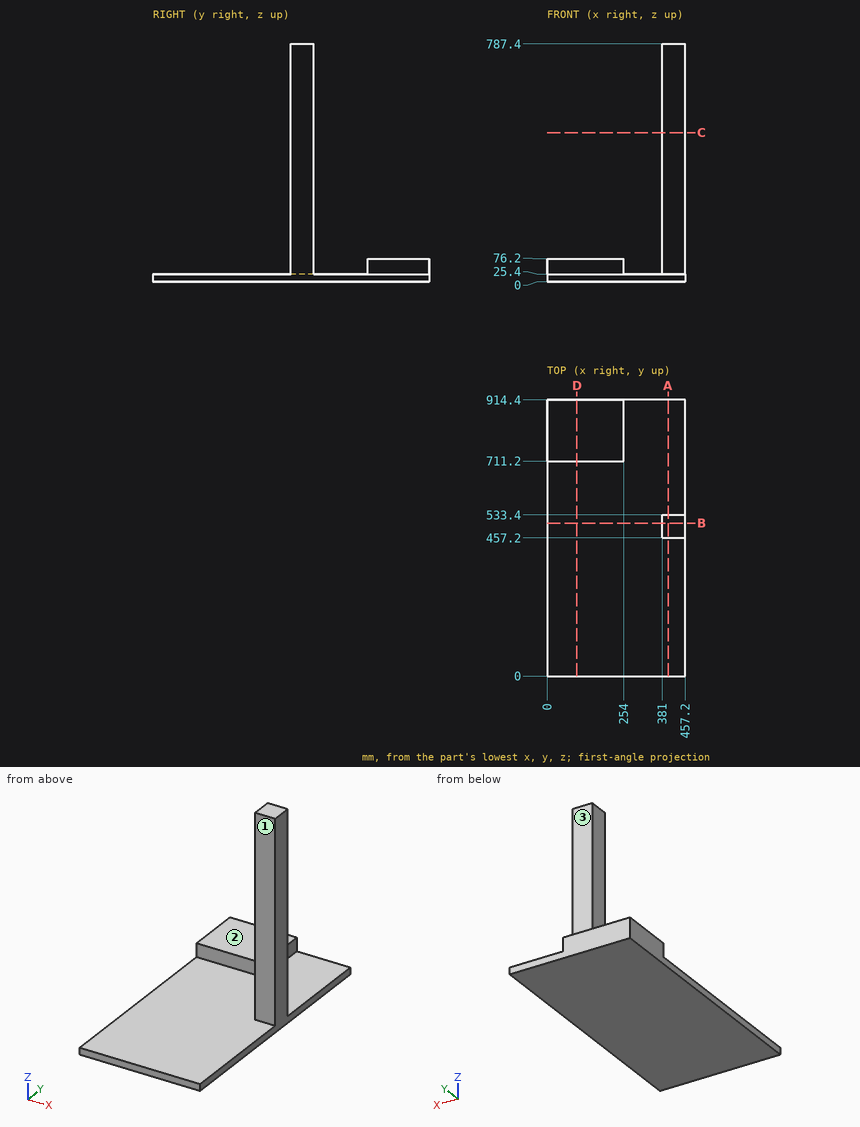
Input: dimensioned drawing with shaded views. Units: mm. Origin: part minimum x, y, z. A direction names the side the tool comes from. Give positions to 0.01 mm unless a question says otherwise; leave off trailing zeros. Order: outer loops, then holes, each group sorted by start corner. A loop starts at its lowest first (then second) coordinate and runs counter-clockwise, first axis right, second up. Notation, with made-up numbers: (-11, -28.75) -> (8, -28.75) arc R32 cw to (8, 0.25) -> close; hole circle Ø6 at (71, 26). An arc over 180 degrees is marked (long way). Answer as a JSON object with one key per item and string values.
Q1. Section B-B (y = 506). Output: boundary loops of the cut face in (x, z), plus the area to 3 significant figures.
Entries:
{"outline": "(0, 0) -> (457.2, 0) -> (457.2, 787.4) -> (381, 787.4) -> (381, 25.4) -> (0, 25.4) -> close", "area": "69,700 mm^2"}
Q2. First-contact query: pin 1 (3 mm diameter, centred on x = 403.5, z = 507, fed in from +Y); pin 2 (5 mm diameter, centred on y = 534.5, z = 233.5, fed in from -X); pin 3 (5 mm diameter, centred on x = 397.5, y = 425.5, fed in from +Z). Flat tips, straight axial feed; report the tip coordinate or a pass-through.
Entries:
{"pin 1": "stops at y = 533.4", "pin 2": "stops at x = 381", "pin 3": "stops at z = 25.4"}
Q3. Section C-C (z = 494). Output: boundary loops of the cut face in (x, y).
Entries:
{"outline": "(381, 457.2) -> (457.2, 457.2) -> (457.2, 533.4) -> (381, 533.4) -> close"}
Q4. Section A-A (x = 400.5). Output: boundary loops of the cut face in (y, z), plus the area to 3 significant figures.
Entries:
{"outline": "(0, 0) -> (914.4, 0) -> (914.4, 25.4) -> (533.4, 25.4) -> (533.4, 787.4) -> (457.2, 787.4) -> (457.2, 25.4) -> (0, 25.4) -> close", "area": "81,300 mm^2"}
Q5. Material intervals for probe 1 along Z at (x, y) = (224, 316.5); probe 2 along Y at (x, z) = (416, 369.5); probe 3 along Z at (x, y) = (248.5, 780.5), sorted ascending.
Entries:
{"probe 1": "z = 0 to 25.4", "probe 2": "y = 457.2 to 533.4", "probe 3": "z = 0 to 76.2"}
Q6. Access query for the marked faces 1, 2 and 3. Directions: +Z, -Z, +X, -X, +Y, -Y. A direction counts if a zero-diameter tool reaches every point of the face in a straight line with its end or side. Return the directions, or none.
Entries:
{"face 1": "+Z, +X, -X, -Y", "face 2": "+Z, +X, -X, +Y, -Y", "face 3": "+Z, +X, -X, +Y"}
Q7. Section D-D (x = 98.5). Output: boundary loops of the cut face in (y, z), plus the area to 3 significant figures.
Entries:
{"outline": "(0, 0) -> (914.4, 0) -> (914.4, 76.2) -> (711.2, 76.2) -> (711.2, 25.4) -> (0, 25.4) -> close", "area": "33,500 mm^2"}
